Geometry: final body of the model. Coordinates: model frame, mm. Face numbers are marked on the shaded views. Give positions to 0.01 mm unless a question says otherwise; leave off trailing zeros. Loops run counter-clockwise (first coordinate to the right, second up) from the corner with the lowest first, then second, coordinate; pieces in that order, holes last. Notation, with made-up numbers: (-12, 88) -> (23, 88) arc R24 ccw to (23, 113) -> close; hole circle Ø3 at (75, 34). An arc over 180 degrees is marked (long way). One line per question, with ' | ' between items. Start each with the question number.
Item 1: Mould query, pull axis Y, two halves, no side actions, for the marked faces 1, 2 and 3. Classes: released by +Y, released by -Y, zero draft, split by the parting line, or undercut.
Item 2: Section A-A on y = -460. Give the number of separate pieces and of enclosed holes in the cut face, then the cut area to 3 significant figures.
Item 3: Section B-B on y = -402. Return loops of the section in (x, z).
Item 4: Material intervals for line 1 along X through (y, z) = (-210.5, 13.5); line 2 along X through (y, z) = (-444.5, 50); line 3 along Z through (x, y) = (-138.5, -163.5), sorted ascending. Write a range as [from, to].
Item 5: Section C-C on x = -107. Return loops of the section in (y, z), then the cut area to 3 significant figures.
Item 6: Pin query (flat end, axial travel): P1, Ø1, axis at x = -191.5, z = 59, coming from the +Y side; P2, Ø5, axis at x = -227, z = 20.5, coming from the -Y side. Return the tip coordinate at first contact, or that it passes through.
from build123d import *

# Parameters (mm, degrees)
F0_W      = 20
F0_H      = 20
F1_DEPTH  = 500
F2_W      = 20
F2_H      = 20
F3_DEPTH  = 470
F4_W      = 20
F4_H      = 20
F5_DEPTH  = 460
F6_W      = 20
F6_H      = 20
F7_DEPTH  = 110
F8_W      = 20
F8_H      = 20
F9_DEPTH  = 160
F10_W     = 20
F10_H     = 20
F10_H_2   = 130
F11_DEPTH = 40
F13_W     = 160
F13_H     = 20
F14_DEPTH = 120.001
F16_D     = 20
F16_DEPTH = 250
F16_TIP   = 6.0086061903
F17_W     = 160
F17_H     = 80
F18_DEPTH = 20
F19_W     = 20
F19_H     = 20
F20_DEPTH = 350


with BuildPart() as f1:
    # F0 (on Front) → F1 (new body)
    with BuildSketch(Plane.XZ):
        with Locations((10, 10)):
            Rectangle(F0_W, F0_H)
    extrude(amount=F1_DEPTH)

    # F2 (on face) → F3 (join)
    with BuildSketch(Plane(origin=(0, 0, 0), x_dir=(0, -1, 0), z_dir=(-1, 0, 0))):
        with Locations((10, 10)):
            Rectangle(F2_W, F2_H)
        with Locations((490, 10)):
            Rectangle(F2_W, F2_H)
    extrude(amount=F3_DEPTH)

    # F4 (on face) → F5 (join, through all)
    with BuildSketch(Plane.XZ.offset(20)):
        with Locations((-460, 10)):
            Rectangle(F4_W, F4_H)
    extrude(amount=F5_DEPTH)

    # F6 (on face) → F7 (join)
    with BuildSketch(Plane(origin=(0, -480, 0), x_dir=(-1, 0, 0), z_dir=(0, 1, 0))):
        with Locations((135, 10)):
            Rectangle(F6_W, F6_H)
        with Locations((315, 10)):
            Rectangle(F6_W, F6_H)
    extrude(amount=F7_DEPTH)

    # F8 (on face) → F9 (join, through all)
    with BuildSketch(Plane(origin=(-145, 0, 0), x_dir=(0, -1, 0), z_dir=(-1, 0, 0))):
        with Locations((380, 10)):
            Rectangle(F8_W, F8_H)
    extrude(amount=F9_DEPTH)

    # F10 (on face) → F11 (join)
    with BuildSketch(Plane.XY.offset(20)):
        with Locations((-460, -490)):
            Rectangle(F10_W, F10_H)
        with Locations((10, -490)):
            Rectangle(F10_W, F10_H)
        with Locations((-460, -10)):
            Rectangle(F10_W, F10_H)
        with Locations((10, -10)):
            Rectangle(F10_W, F10_H)
        with Locations((10, -250)):
            Rectangle(F10_W, F10_H)
        with Locations((-460, -250)):
            Rectangle(F10_W, F10_H)
        with Locations((-315, -435)):
            Rectangle(F10_W, F10_H_2)
        with Locations((-135, -435)):
            Rectangle(F10_W, F10_H_2)
        with Locations((-225, -10)):
            Rectangle(F10_W, F10_H)
    extrude(amount=F11_DEPTH)

    # F12: F1 across face


with BuildPart() as f1_1:
    add(f1.part)
    add(f1.part.mirror(Plane(origin=(10, -10, 60), x_dir=(1, 0, 0), z_dir=(0, 0, 1))))

    # F13 (on face) → F14 (cut, through all)
    with BuildSketch(Plane.XY.offset(120)):
        with Locations((-225, -490)):
            Rectangle(F13_W, F13_H)
    extrude(amount=-F14_DEPTH, mode=Mode.SUBTRACT)

    # F16
    with Locations(Plane.YZ.offset(-125)):
        with Locations((-460, 60)):
            Hole(F16_D / 2, depth=F16_DEPTH)
            with Locations((0, 0, -(F16_DEPTH + F16_TIP / 2))):  # 118° drill point
                Cone(0, F16_D / 2, F16_TIP, mode=Mode.SUBTRACT)

    # F17 (on face) → F18 (join)
    with BuildSketch(Plane(origin=(0, -370, 0), x_dir=(-1, 0, 0), z_dir=(0, 1, 0))):
        with Locations((225, 60)):
            Rectangle(F17_W, F17_H)
    extrude(amount=-F18_DEPTH)

    # F19 (on face) → F20 (join, through all)
    with BuildSketch(Plane(origin=(0, -370, 0), x_dir=(-1, 0, 0), z_dir=(0, 1, 0))):
        with Locations((135, 10)):
            Rectangle(F19_W, F19_H)
        with Locations((315, 10)):
            Rectangle(F19_W, F19_H)
        with Locations((315, 110)):
            Rectangle(F19_W, F19_H)
        with Locations((135, 110)):
            Rectangle(F19_W, F19_H)
    extrude(amount=F20_DEPTH)


solid = f1_1.part
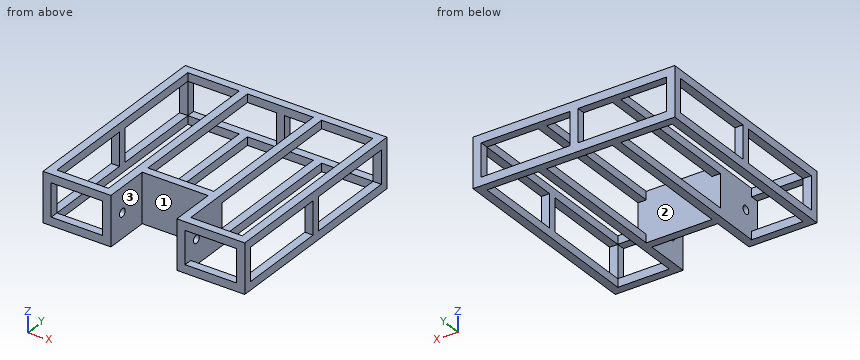
Result sheet:
1) face 1: released by -Y | face 2: undercut | face 3: zero draft
2) separate pieces: 8 | enclosed holes: 0 | area: 5,600 mm²
3) outline: (-470, 0) -> (-450, 0) -> (-450, 20) -> (-470, 20) -> close; (-470, 100) -> (-450, 100) -> (-450, 120) -> (-470, 120) -> close; (-325, 0) -> (-305, 0) -> (-305, 120) -> (-325, 120) -> close; (-145, 0) -> (-125, 0) -> (-125, 120) -> (-145, 120) -> close; (0, 0) -> (20, 0) -> (20, 20) -> (0, 20) -> close; (0, 100) -> (20, 100) -> (20, 120) -> (0, 120) -> close
4) line 1: x = [-470, -450], [-325, -305], [-145, -125], [0, 20] | line 2: x = [-325, -305], [-145, -125] | line 3: z = [0, 20], [100, 120]
5) outline: (-500, 0) -> (-480, 0) -> (-480, 20) -> (-500, 20) -> close; (-500, 100) -> (-480, 100) -> (-480, 120) -> (-500, 120) -> close; (-20, 0) -> (0, 0) -> (0, 20) -> (-20, 20) -> close; (-20, 100) -> (0, 100) -> (0, 120) -> (-20, 120) -> close | area: 1,600 mm²
6) P1: stops at y = -370 | P2: stops at y = -390
